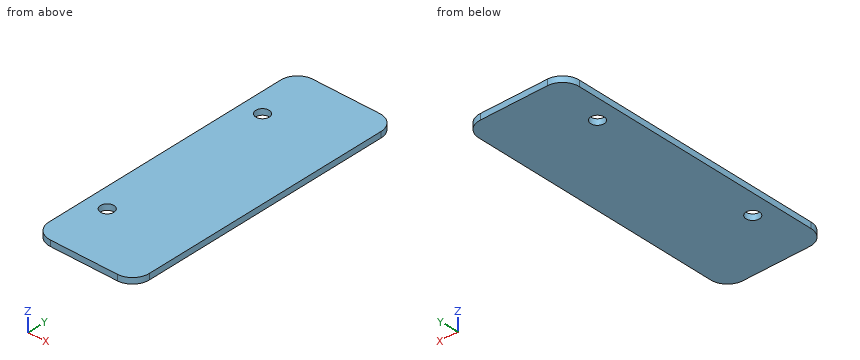
from build123d import *

# Parameters (mm, degrees)
SKETCH_1_W          = 60
SKETCH_1_H          = 171.5
EXTRUDE_1_DEPTH     = 3.5
FILLET_1_R          = 10
CUT_EXTRUDE_1_REACH = 5.5
SKETCH_2_R          = 4


with BuildPart() as part:
    # 草图1 → 凸台-拉伸1 (new body)
    with BuildSketch(Plane.XY):
        with Locations((2332, -8)):
            Rectangle(SKETCH_1_W, SKETCH_1_H)
    extrude(amount=EXTRUDE_1_DEPTH)

    # 圆角1
    fillet_1_edges = [part.edges().sort_by_distance(p)[0] for p in [
        (2302, -93.75, 1.75),
        (2302, 77.75, 1.75),
        (2362, 77.75, 1.75),
        (2362, -93.75, 1.75),
    ]]
    fillet(fillet_1_edges, radius=FILLET_1_R)

    # 草图2 → 切除-拉伸1 (cut, up to next)
    with BuildSketch(Plane.XY.offset(3.5), mode=Mode.PRIVATE) as cut_extrude_1_sk1:
        with Locations((2314, 42.75)):
            Circle(SKETCH_2_R)
    cut_extrude_1_tool1 = extrude(cut_extrude_1_sk1.sketch, amount=-CUT_EXTRUDE_1_REACH, mode=Mode.PRIVATE) & part.part
    add(cut_extrude_1_tool1.solids().sort_by_distance((2314, 42.75, 3.5))[0], mode=Mode.SUBTRACT)
    # 草图2 → 切除-拉伸1 (cut, up to next)
    with BuildSketch(Plane.XY.offset(3.5), mode=Mode.PRIVATE) as cut_extrude_1_sk2:
        with Locations((2314, -58.75)):
            Circle(SKETCH_2_R)
    cut_extrude_1_tool2 = extrude(cut_extrude_1_sk2.sketch, amount=-CUT_EXTRUDE_1_REACH, mode=Mode.PRIVATE) & part.part
    add(cut_extrude_1_tool2.solids().sort_by_distance((2314, -58.75, 3.5))[0], mode=Mode.SUBTRACT)


solid = part.part
Can you work these out from the model? Positions are in its coordinate system, mm. Coordinates: 2 decimals unless noted, no trailing zeros. Write each loop counter-clockwise with the first axis right and the second up, starting at its lowest first coordinate (ties: lowest second). Pieces come first, ordered by that corner, then holes. Notation, with made-up numbers: (80, -10) -> (96, -10) arc R24 cw to (96, 2) -> close; hole circle Ø4 at (70.25, 11.25). An arc over 180 degrees is marked (long way). Write each question's results on one line, items separated by ' | '. Start each with the question number.
Q1. Imagine slicing it at A-A (x = 2314). Write out the boundary of the cut face in (y, z).
Q2. If I drill on probe 1 along Y at (x, z) = (2314, 2.85); probe 2 along Y at (x, z) = (2315, 3.2); probe 3 along X at (y, z) = (42, 2.25), over which ranges is the centre line in solid material (lowest first)?
Q3. Imagine slicing it at C-C (z = 0.55). Write out the boundary of the cut face in (x, y).
Q4. Imagine slicing it at B-B (y = -58.75). Write out the boundary of the cut face in (x, z).
Taken from the geometry:
1) outline: (-93.75, 0) -> (-62.75, 0) -> (-62.75, 3.5) -> (-93.75, 3.5) -> close; (-54.75, 0) -> (38.75, 0) -> (38.75, 3.5) -> (-54.75, 3.5) -> close; (46.75, 0) -> (77.75, 0) -> (77.75, 3.5) -> (46.75, 3.5) -> close
2) probe 1: y = -93.75 to -62.75, -54.75 to 38.75, 46.75 to 77.75 | probe 2: y = -93.75 to -62.62, -54.88 to 38.88, 46.62 to 77.75 | probe 3: x = 2302 to 2310.07, 2317.93 to 2362
3) outline: (2302, -83.75) arc R10 ccw to (2312, -93.75) -> (2352, -93.75) arc R10 ccw to (2362, -83.75) -> (2362, 67.75) arc R10 ccw to (2352, 77.75) -> (2312, 77.75) arc R10 ccw to (2302, 67.75) -> close; hole circle Ø8 at (2314, -58.75); hole circle Ø8 at (2314, 42.75)
4) outline: (2302, 0) -> (2310, 0) -> (2310, 3.5) -> (2302, 3.5) -> close; (2318, 0) -> (2362, 0) -> (2362, 3.5) -> (2318, 3.5) -> close
